Part model, mm, in its own coordinate system. A direction names the side the tool comes from. Round coordinates to 2 decimals unless told otherwise and drop trailing zeros. Write each loop counter-clockwise with the first axis right and the second up, starting at its lowest first coordinate (ties: lowest second). Pieces come first, ordered by that corner, then holes.
```python
from build123d import *

# Parameters (mm, degrees)
SKETCH5_W           = 20
SKETCH5_H           = 20
BOSS_EXTRUDE1_DEPTH = 10
SKETCH6_R           = 2.5
BOSS_EXTRUDE2_DEPTH = 5
FILLET1_R           = 5
SHELL2_T            = -2


with BuildPart() as part:
    # Sketch5 → Boss-Extrude1 (new body)
    with BuildSketch(Plane(origin=(0, 0, 0), x_dir=(0, 0, -1), z_dir=(1, 0, 0))):
        with Locations((10, 10)):
            Rectangle(SKETCH5_W, SKETCH5_H)
    extrude(amount=BOSS_EXTRUDE1_DEPTH)

    # Sketch6 → Boss-Extrude2 (add)
    with BuildSketch(Plane(origin=(10, 0, 0), x_dir=(0, 0, -1), z_dir=(1, 0, 0))):
        with Locations(Location((5, 15, 0), (0, 0, 180))):
            Circle(SKETCH6_R)
        with Locations(Location((15, 15, 0), (0, 0, 180))):
            Circle(SKETCH6_R)
        with Locations(Location((15, 5, 0), (0, 0, 180))):
            Circle(SKETCH6_R)
        with Locations(Location((5, 5, 0), (0, 0, 180))):
            Circle(SKETCH6_R)
    extrude(amount=BOSS_EXTRUDE2_DEPTH)

    # Fillet1
    fillet1_edges = [part.edges().sort_by_distance(p)[0] for p in [
        (5, 20, 0),
        (5, 20, -20),
        (5, 0, -20),
        (5, 0, 0),
    ]]
    fillet(fillet1_edges, radius=FILLET1_R)

    # Shell2
    shell2_openings = [part.faces().sort_by_distance(p)[0] for p in [
        (0, 10, -10),
    ]]
    offset(amount=SHELL2_T, openings=shell2_openings, kind=Kind.INTERSECTION)


solid = part.part
```
Q1. Drop flat-ended pins along their axis: pin 1 (1.1 mm diameter, centred on y = 15, z = -15, fed in from -X); pin 2 (0.5 mm diameter, centred on y = 5, z = -5, fed in from -X); pin 3 (4 mm diameter, centred on x = 13, y = 6.5, fed in from +Z); pin 4 (1.5 mm diameter, centred on x = 11, z = -9, fed in from -Y). Give the stop position or say it passes through.
Values follow:
pin 1: stops at x = 8
pin 2: stops at x = 13
pin 3: stops at z = -2.5
pin 4: passes through
Q2. Cut at B-B on z = -13.5. Write the cut outline in (x, y), plus the area to 3 significant figures.
Values follow:
outline: (0, 0) - (10, 0) - (10, 3) - (15, 3) - (15, 7) - (10, 7) - (10, 13) - (15, 13) - (15, 17) - (10, 17) - (10, 20) - (0, 20) - (0, 18) - (8, 18) - (8, 2) - (0, 2) - close
area: 112 mm2
Q3. Cut at A-A on x = 11. Write the cut outline in (y, z), plus the area to 3 significant figures.
Values follow:
outline: circle Ø5 at (5, -15); circle Ø5 at (5, -5); circle Ø5 at (15, -15); circle Ø5 at (15, -5); hole circle Ø1 at (5, -15); hole circle Ø1 at (5, -5); hole circle Ø1 at (15, -15); hole circle Ø1 at (15, -5)
area: 75.4 mm2
Q4. Cut at D-D on z = -8.75. Write the cut outline in (x, y), plus the area to 3 significant figures.
Values follow:
outline: (0, 0) - (10, 0) - (10, 20) - (0, 20) - (0, 18) - (8, 18) - (8, 2) - (0, 2) - close
area: 72.0 mm2
Q5. Which spindle directions (+Z, -Z, +X, -X, +Y, -Y) get a long thin tool onto all of the face, cutting with end or side? Do faces 1 (the cylindrical face through (4.06, 2.86, -17.1)), 2 (the flat face through (5, 20, -10)), 3 (the cylindrical face through (12.465, 4.249, -2.615)). Say none if no direction does.
Values follow:
face 1: -X
face 2: +Z, -Z, +X, -X, +Y
face 3: +X
Q6. Wall check: L1, parallel to Y at x = 9.6, z = -15; L2, parallel to Z at x = 7, y = 9; L3, parallel to Y at x = 3.75, z = -9.75. Give the ranges that are in metal, low to high.
Values follow:
L1: y = 0 to 4.5, 5.5 to 14.5, 15.5 to 20
L2: z = -20 to -18, -2 to 0
L3: y = 0 to 2, 18 to 20
Q7. Cut at C-C on x = 7.25. Write the cut outline in (y, z), plus the area to 3 significant figures.
Values follow:
outline: (0, -15) arc R5 ccw to (5, -20) - (15, -20) arc R5 ccw to (20, -15) - (20, -5) arc R5 ccw to (15, 0) - (5, 0) arc R5 ccw to (0, -5) - close; hole (2, -15) arc R3 ccw to (5, -18) - (15, -18) arc R3 ccw to (18, -15) - (18, -5) arc R3 ccw to (15, -2) - (5, -2) arc R3 ccw to (2, -5) - close
area: 130 mm2
Q8. Mould opens along Y. For faces 4 (the flat face through (4, 10, -18)), 5 (the flat face through (5, 0, -10)), 6 (the flat face through (0, 9.3, -1.8)) say: +Y half, -Y half, draft (parallel to the pull), parting line (faces both ways), or undercut.
Values follow:
face 4: undercut
face 5: -Y half
face 6: draft
